Autodesk Inventor part; units mm, degrees
ref_plane "YZ Plane" through (0, 0, 0) normal (1, 0, 0) x (0, 1, 0)
ref_plane "XZ Plane" through (0, 0, 0) normal (0, 1, 0) x (-1, 0, 0)
ref_plane "XY Plane" through (0, 0, 0) normal (0, 0, 1) x (1, 0, 0)
sketch "Sketch1" plane through (0, 0, 0) normal (0, 0, 1) x (1, 0, 0)
  line L0 (0, 0) -> (-25.4, 0)
  line L1 (-25.4, 0) -> (-25.4, 25.4)
  line L2 (-25.4, 25.4) -> (0, 25.4)
  line L3 (0, 25.4) -> (0, 0)
  line L4 (-3.175, 22.225) -> (-22.225, 22.225)
  line L5 (-22.225, 22.225) -> (-22.225, 3.175)
  line L6 (-22.225, 3.175) -> (-3.175, 3.175)
  line L7 (-3.175, 3.175) -> (-3.175, 22.225)
  dimension "d0" = 25.4
  dimension "d2" = 25.4
  dimension "d3" = 3.175
extrude "Extrusion1" add sketch "Sketch1" along normal blind 660.4
sketch "Sketch2" plane through (0, 0, 0) normal (1, 0, 0) x (0, 0, -1)
  line L0 (0, 25.4) -> (0, 0)
  line L1 (0, 25.4) -> (-660.4, 25.4)
  line L2 (-660.4, 0) -> (-660.4, 25.4)
  line L3 (0, 0) -> (-660.4, 0)
  line L4 (-113.1604, 25.4) -> (-351.652, -111.264)
  line L5 (-351.652, -111.264) -> (-415.4102, 0)
  line L6 (-113.1604, 0) -> (0, 0)
  line L7 (-113.1604, 25.4) -> (0, 25.4)
  line L8 (0, 25.4) -> (0, 0)
  line L9 (-444.6849, 0) -> (-660.4, 0)
  line L10 (-660.4, 0) -> (-660.4, 25.4)
  line L11 (-660.4, 25.4) -> (-429.9653, 25.4)
  line L12 (-429.9653, 25.4) -> (-415.4102, 0)
  line L13 (-113.1604, 25.4) -> (-100.5318, 3.3619)
  line L14 (-100.5318, 3.3619) -> (-361.0615, -145.9308)
  line L15 (-361.0615, -145.9308) -> (-444.6849, 0)
  dimension "d6" = 25.4
  dimension "d9" = 25.4
  dimension "d12" = 25.4
properties part number "bar"
Input: part model. Units: mm. Frame: model coordinates. A direction names the side the tool comes from. Round coordinates to 2 decimals unless told otherwise and drop trailing zeros. Loops run counter-clockwise (first coordinate to the right, second up) from the corner with the lowest first, then second, coordinate; pieces in that order, holes last. Notation, with made-up numbers: (64, 16) -> (88, 16) arc R22 cw to (88, 28) -> close; hole circle Ø8 at (88, 5.5). An arc over 180 degrees is marked (long way). Answer as a JSON object with one key per item and string values. Group by question number.
1) Ray query, L1, parallel to Y at x = -15.5, z = 585.5 (3 decimals); L2, parallel to X at y = 5, z = 300.5 (3 decimals). Return the intervals inside material, ascending.
2) Reachability of faces 5 (the flat face through (-3.175, 13, 326)), 6 (the flat face through (-13, 0, 326)) from +Z, -Z, +X, -X, +Y, -Y: full face, straight path, thin tool, end or side. Return the list, or none.
3) Section query C-C on z = 157. Output: boundary loops of the cut face in (x, y) (3 decimals).
4) Draft query along X for faces 1 (the flat face through (-13, 22.225, 326)), 2 (the flat face through (-2, 13, 0)), 3 (the flat face through (0, 13, 326)), 4 (the flat face through (-25.4, 13, 326)). Return one class per face: +X half, -X half, draft (parallel to the pull), parting line (faces both ways), or undercut.
5) Section query A-A on y = 15. Output: boundary loops of the cut face in (x, z) (3 decimals), plus the area to 3 significant figures.
6) Section query B-B on x = -16. Output: boundary loops of the cut face in (y, z) (3 decimals), plus the area to 3 significant figures.
Reply:
{
 "1": {"L1": "y = 0 to 3.175, 22.225 to 25.4", "L2": "x = -25.4 to -22.225, -3.175 to 0"},
 "2": {"face 5": "+Z, -Z", "face 6": "+Z, -Z, +X, -X, -Y"},
 "3": {"outline": "(-25.4, 0) -> (0, 0) -> (0, 25.4) -> (-25.4, 25.4) -> close; hole (-22.225, 3.175) -> (-3.175, 3.175) -> (-3.175, 22.225) -> (-22.225, 22.225) -> close"},
 "4": {"face 1": "undercut", "face 2": "draft", "face 3": "+X half", "face 4": "-X half"},
 "5": {"outline": "(-25.4, 0) -> (-22.225, 0) -> (-22.225, 660.4) -> (-25.4, 660.4) -> close; (-3.175, 0) -> (0, 0) -> (0, 660.4) -> (-3.175, 660.4) -> close", "area": "4,190 mm2"},
 "6": {"outline": "(0, 0) -> (3.175, 0) -> (3.175, 660.4) -> (0, 660.4) -> close; (22.225, 0) -> (25.4, 0) -> (25.4, 660.4) -> (22.225, 660.4) -> close", "area": "4,190 mm2"}
}
